Part model, mm, in its own coordinate system. Give positions to 0.01 mm unless a question says otherwise; leave off trailing zeros. Order: outer loops, then holes, each group sorted by start corner. A loop starts at its lowest first (then second) coordinate and runs counter-clockwise, first axis right, second up. Notation, with made-up numbers: (-18.5, 58.25) - (35.5, 58.25) arc R15 ccw to (35.5, 73.25) - close; hole circle Ø11 at (79.25, -13.75). An arc over 180 degrees is marked (long way). Use one line per item in the form item = value. Start each with the question number.
1. Band-saw the part on C-C, the plane y = 17.5. List the corners of the cut face in (x, z), plus the area to 3 significant figures.
2. Band-saw the part on B-B, the plane z = 0.55. List the corners of the cut face in (x, y), plus the area to 3 significant figures.
3. Band-saw the part on A-A, the plane x = -8.5. List the corners of the cut face in (y, z), plus the area to 3 significant figures.
4. Drill centre lines: line 1 (X direction, y = 10, z = 0.65); line 2 (Y direction, x = -8, z = 0.3); line 3 (Y direction, x = -17.25, z = 0.3). Where is each one in solid material? Low to high.
Autodesk Inventor part; units mm, degrees
ref_plane "YZ Plane" through (0, 0, 0) normal (1, 0, 0) x (0, 1, 0)
ref_plane "XZ Plane" through (0, 0, 0) normal (0, 1, 0) x (-1, 0, 0)
ref_plane "XY Plane" through (0, 0, 0) normal (0, 0, 1) x (1, 0, 0)
sketch "Sketch1" plane through (0, 0, 0) normal (0, 0, 1) x (1, 0, 0)
  line L0 (0, -23) -> (0, 23)
  line L1 (0, -23) -> (-25, 0)
  line L2 (-25, 0) -> (0, 23)
  point P0 (0, 0)
  point P1 (0, 0)
  point P2 (0, 0)
  dimension "d1" = 46
  dimension "d9" = 25
extrude "Plate1" add sketch "Sketch1" along normal blind 0.8
fillet "Corner Round2" radius 1 3 edges at (0, -23, 0.4) (-25, 0, 0.4) (0, 23, 0.4)
equation "\"d2\" = Thickness"
equation "\"BendReliefWidth\" = Thickness"
equation "\"BendReliefDepth\" = 0.5 * Thickness"
equation "\"CornerReliefSize\" = 4 * Thickness"
equation "\"MinimumRemnant\" = 2 * Thickness"
equation "\"TransitionRadius\" = BendRadius"
equation "\"JacobiRadiusSize\" = BendRadius"
equation "\"GapSize\" = Thickness"
properties part number "DS-B-503 CAP" material "Stainless Steel"
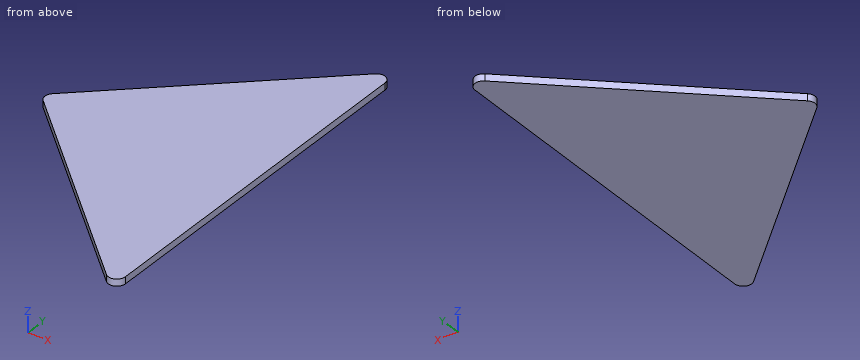
From the geometry:
q1.outline = (-5.98, 0) - (0, 0) - (0, 0.8) - (-5.98, 0.8) - close
q1.area = 4.78 mm²
q2.outline = (-24.2, -0.74) - (-1.68, -21.46) arc R1 ccw to (0, -20.72) - (0, 20.72) arc R1 ccw to (-1.68, 21.46) - (-24.2, 0.74) arc R1 ccw to start
q2.area = 572 mm²
q3.outline = (-15.18, 0) - (15.18, 0) - (15.18, 0.8) - (-15.18, 0.8) - close
q3.area = 24.3 mm²
q4.line_1 = -14.13 to 0
q4.line_2 = -15.64 to 15.64
q4.line_3 = -7.13 to 7.13
